Input: part model. Units: mm. Frame: model coordinates. A direction names the side the tool comes from. Round coordinates to 2 decimals unless told otherwise and drop trailing zeros. Loops run counter-clockwise (first coordinate to the right, second up) from the corner with the lowest first, then second, coordinate; pieces in that order, holes last. Notation, with made-up numbers: (25.5, 26) - (78.5, 26) arc R21 ccw to (78.5, 40) - close; hole circle Ø3 at (70.5, 89). An arc over 180 degrees is marked (long way). One line per question, with ' | ' between items. Start each with the question number.
from build123d import *

# Parameters (mm, degrees)
F0_R      = 19.71
F1_DEPTH  = 7.6
F2_W      = 40
F2_H      = 7.75
F3_DEPTH  = 4.7
F4_W      = 7.55
F4_H      = 13.75
F5_DEPTH  = 4.7
F6_W      = 8.35
F6_H      = 5.3
F7_DEPTH  = 3.6
F8_W      = 2.175
F8_H      = 1.2
F9_DEPTH  = 3.601
F10_R     = 3.25
F11_DEPTH = 3


with BuildPart() as f1:
    # F0 (on Top) → F1 (new body)
    with BuildSketch(Plane.XY):
        Circle(F0_R)
    extrude(amount=F1_DEPTH)

    # F2 (on face) → F3 (cut)
    with BuildSketch(Plane.XY.offset(7.6)):
        with Locations((0, -0.025)):
            Rectangle(F2_W, F2_H)
    extrude(amount=-F3_DEPTH, mode=Mode.SUBTRACT)

    # F4 (on face) → F5 (cut)
    with BuildSketch(Plane.XY.offset(7.6)):
        Rectangle(F4_W, F4_H)
    extrude(amount=-F5_DEPTH, mode=Mode.SUBTRACT)

    # F6 (on face) → F7 (join)
    with BuildSketch(Plane(origin=(0, 0, 0), x_dir=(1, 0, 0), z_dir=(0, 0, -1))):
        with Locations((0, -21.987913)):
            Rectangle(F6_W, F6_H)
    extrude(amount=-F7_DEPTH)

    # F8 (on face) → F9 (cut, through all)
    with BuildSketch(Plane.XY.offset(3.6)):
        Polygon((2, 22.937913), (-2, 22.937913), (-2, 19.837913), (2, 19.837913), (2, 20.219285), (2, 21.419285), align=None)
        with Locations((3.0875, 20.819285)):
            Rectangle(F8_W, F8_H)
    extrude(amount=-F9_DEPTH, mode=Mode.SUBTRACT)

    # F10 (on face) → F11 (cut)
    with BuildSketch(Plane(origin=(0, 0, 0), x_dir=(1, 0, 0), z_dir=(0, 0, -1))):
        Circle(F10_R)
    extrude(amount=-F11_DEPTH, mode=Mode.SUBTRACT)


solid = f1.part
(1) Line query: line 1 along Y through (x, z) = (0, 1.3); line 2 along X through (y, z) = (0, 1.8); line 3 along Z through (x, y) = (-11.5, -3.5). Output: solid intervals per line, ascending. Write a range as from..to.
(2) Section C-C, the plane z = 1.25. Output: boundary loops of the cut face in (x, y) (3 decimals).
(3) Section B-B, the plane y = 0. Output: boundary loops of the cut face in (x, z).
(4) Reachability of faces 1 (the face through (-2, 21, 2)), 2 (the face through (-3.775, -5, 5)), 3 (the face through (3, 21.419, 2)), 4 (the face through (4.175, 23, 2)) from +Z, -Z, +X, -X, +Y, -Y: full face, straight path, thin tool, end or side. Return the list, or none.
(5) Section D-D, the plane x = -16. Output: boundary loops of the cut face in (y, z), plus the area to 3 significant figures.
(6) Pin query (flat end, axial travel): P1, Ø3, axis at x = 1, z = 5.5, coming from the +Y side; P2, Ø2.5, axis at y = 5, z = 4, coming from the -X side; P3, Ø1, axis at x = 9, z = 4, coming from the -Y side. Return the tip coordinate at first contact, or that it passes through.
(7) Pull-direction query (Y, two-part tool) for faces 5 (the face through (3.775, -5, 5)), 6 (the face through (0, 24.638, 2)), 7 (the face through (-3.775, 5, 5)), 8 (the face through (-0.1, 23.1, 3.6)); classes: released by +Y, released by -Y, zero draft, split by the parting line, or undercut.
(8) Section A-A, the plane x = 0. Output: boundary loops of the cut face in (y, z) (3 decimals), plus the area to 3 significant figures.
Derived:
1) line 1: y = -19.71..-3.25, 3.25..19.84, 22.94..24.64 | line 2: x = -19.71..-3.25, 3.25..19.71 | line 3: z = 0..2.9
2) outline: (-4.175, 19.338) - (-3.812, 19.338) arc R19.71 ccw (long way) to (3.812, 19.338) - (4.175, 19.338) - (4.175, 20.219) - (2, 20.219) - (2, 19.838) - (-2, 19.838) - (-2, 22.938) - (2, 22.938) - (2, 21.419) - (4.175, 21.419) - (4.175, 24.638) - (-4.175, 24.638) - close; hole circle Ø6.5 at (0, 0)
3) outline: (-19.71, 0) - (-3.25, 0) - (-3.25, 2.9) - (-19.71, 2.9) - close; (3.25, 0) - (19.71, 0) - (19.71, 2.9) - (3.25, 2.9) - close
4) face 1: +Z, -Z | face 2: +Z | face 3: +Z, -Z, +X | face 4: +Z, -Z, +X, +Y
5) outline: (-11.51, 0) - (11.51, 0) - (11.51, 7.6) - (3.85, 7.6) - (3.85, 2.9) - (-3.9, 2.9) - (-3.9, 7.6) - (-11.51, 7.6) - close | area: 139 mm²
6) P1: stops at y = 19.71 | P2: stops at x = -19.33 | P3: stops at y = -17.78
7) face 5: undercut | face 6: released by +Y | face 7: undercut | face 8: zero draft
8) outline: (-19.71, 0) - (-3.25, 0) - (-3.25, 2.9) - (-6.875, 2.9) - (-6.875, 7.6) - (-19.71, 7.6) - close; (3.25, 0) - (19.838, 0) - (19.838, 3.6) - (19.71, 3.6) - (19.71, 7.6) - (6.875, 7.6) - (6.875, 2.9) - (3.25, 2.9) - close; (22.938, 0) - (24.638, 0) - (24.638, 3.6) - (22.938, 3.6) - close | area: 223 mm²
